```python
from build123d import *

# Parameters (mm, degrees)
SKETCH1_W            = 50
SKETCH1_H            = 88
BOSS_EXTRUDE1_DEPTH  = 0.25
BOSS_EXTRUDE2_DEPTH  = 5
SKETCH5_W            = 5
SKETCH5_H            = 11.9
BOSS_EXTRUDE3_DEPTH  = 0.05
CUT_EXTRUDE1_DEPTH   = 0.2
FILLET1_R            = 0.04
FILLET1_OF_MIRROR1_R = 0.04


with BuildPart() as part:
    # Sketch1 → Boss-Extrude1 (new body)
    with BuildSketch(Plane.XY.offset(0.25)):
        with Locations((0, 1.25)):
            Rectangle(SKETCH1_W, SKETCH1_H)
    extrude(amount=-BOSS_EXTRUDE1_DEPTH)

    # Sketch4 → Boss-Extrude2 (add)
    with BuildSketch(Plane(origin=(0, -45.25, 0), x_dir=(-1, 0, 0), z_dir=(0, -1, 0))):
        with BuildLine():
            Line((-26.45, -0.25), (26.45, -0.25))
            ThreePointArc((26.45, -0.25), (26.485355339, -0.235355339), (26.5, -0.2))
            Line((26.5, -0.2), (26.5, 1.4))
            ThreePointArc((26.5, 1.4), (26.485355339, 1.435355339), (26.45, 1.45))
            Line((26.45, 1.45), (20, 1.45))
            Line((20, 1.45), (20, 1.5))
            Line((20, 1.5), (26.5, 1.5))
            ThreePointArc((26.5, 1.5), (26.535355339, 1.485355339), (26.55, 1.45))
            Line((26.55, 1.45), (26.55, -0.25))
            ThreePointArc((26.55, -0.25), (26.535355339, -0.285355339), (26.5, -0.3))
            Line((26.5, -0.3), (-26.5, -0.3))
            ThreePointArc((-26.5, -0.3), (-26.535355339, -0.285355339), (-26.55, -0.25))
            Line((-26.55, -0.25), (-26.55, 1.45))
            ThreePointArc((-26.55, 1.45), (-26.535355339, 1.485355339), (-26.5, 1.5))
            Line((-26.5, 1.5), (-20, 1.5))
            Line((-20, 1.5), (-20, 1.45))
            Line((-20, 1.45), (-26.45, 1.45))
            ThreePointArc((-26.45, 1.45), (-26.485355339, 1.435355339), (-26.5, 1.4))
            Line((-26.5, 1.4), (-26.5, -0.2))
            ThreePointArc((-26.5, -0.2), (-26.485355339, -0.235355339), (-26.45, -0.25))
        make_face()
    boss_extrude2 = extrude(amount=-BOSS_EXTRUDE2_DEPTH)

    # Sketch5 → Boss-Extrude3 (add)
    with BuildSketch(Plane(origin=(0, 0, -1.5), x_dir=(-1, 0, 0), z_dir=(0, 0, -1))):
        with Locations((22.5, -39.3)):
            Rectangle(SKETCH5_W, SKETCH5_H)
        with Locations((-22.5, -39.3)):
            Rectangle(SKETCH5_W, SKETCH5_H)
    boss_extrude3 = extrude(amount=BOSS_EXTRUDE3_DEPTH)

    # Sketch6 → Cut-Extrude1 (cut)
    with BuildSketch(Plane(origin=(0, 0, -1.55), x_dir=(-1, 0, 0), z_dir=(0, 0, -1))):
        Polygon((20, -45.25), (25, -45.25), (20, -40.254912883), align=None)
        Polygon((-20, -40.254912883), (-25, -45.25), (-20, -45.25), align=None)
    cut_extrude1 = extrude(amount=-CUT_EXTRUDE1_DEPTH, mode=Mode.SUBTRACT)

    # Fillet1
    fillet1_edges = [part.edges().sort_by_distance(p)[0] for p in [
        (-22.5, -42.752456442, -1.45),
        (-22.5, -42.752456442, -1.55),
        (22.5, -42.752456442, -1.55),
        (22.5, -42.752456442, -1.45),
    ]]
    fillet(fillet1_edges, radius=FILLET1_R)

    # Mirror1: Boss-Extrude2, Boss-Extrude3, Cut-Extrude1 across plane
    add(boss_extrude2.mirror(Plane(origin=(0, 0, 0), x_dir=(0, 0, 1), z_dir=(0, -1, 0))))
    add(boss_extrude3.mirror(Plane(origin=(0, 0, 0), x_dir=(0, 0, 1), z_dir=(0, -1, 0))))
    add(cut_extrude1.mirror(Plane(origin=(0, 0, 0), x_dir=(0, 0, 1), z_dir=(0, -1, 0))), mode=Mode.SUBTRACT)

    # Fillet1 of Mirror1
    fillet1_of_mirror1_edges = [part.edges().sort_by_distance(p)[0] for p in [
        (-22.5, 42.752456442, -1.45),
        (-22.5, 42.752456442, -1.55),
        (22.5, 42.752456442, -1.55),
        (22.5, 42.752456442, -1.45),
    ]]
    fillet(fillet1_of_mirror1_edges, radius=FILLET1_OF_MIRROR1_R)


solid = part.part
```
Could you check a few things on this model? Use its own coordinates, in mm. Give positions to 0.01 mm unless a question says otherwise; leave off trailing zeros. Order: outer loops, then holes, each group sorted by start corner. A loop starts at its lowest first (then second) coordinate and runs counter-clockwise, first axis right, second up.
Q1. If I drill on line 1 along Z through (x, y) = (2, 16); line 2 along X through (y, z) = (20, 0.1); line 3 along Y through (x, z) = (19, 0.2), over which ranges is the centre line in solid material (lowest first)?
Q2. Suppose I cut it at C-C, the plane x = -6. Write out the boundary of the cut face in (y, z), and give its area (3 significant figures).
Q3. I'm going to push flat-ended pins straight in: P1, Ø1, axis at x = -0.5, y = -32.5, coming from the +Z side; P2, Ø1.2, axis at x = -26, y = 43.5, coming from the -Z side; P3, Ø10, axis at x = 16, y = -8, coming from the -Z side; P4, Ø1.6, axis at x = -25.5, y = -43.5, coming from the -Z side. Where does each tip first touch, or does it pass through?
Q4. Suppose I cut it at A-A, the plane z = -0.45. Write out the boundary of the cut face in (x, y), and give its area (3 significant figures).
Q5. Suppose I cut it at B-B, the plane y = 36.5. Write out the boundary of the cut face in (x, z), and give its area (3 significant figures).
Q6. Suppose I cut it at D-D, the plane x = -21.5. Count the separate pieces of the cut face and the enclosed holes in it, and give its area (3 significant figures).
Solution:
1. line 1: z = 0 to 0.25
1. line 2: x = -25 to 25
1. line 3: y = -42.75 to 45.25
2. outline: (-45.25, 0.25) - (-42.75, 0.25) - (-42.75, 0) - (45.25, 0) - (45.25, 0.3) - (40.25, 0.3) - (40.25, 0.25) - (-40.25, 0.25) - (-40.25, 0.3) - (-45.25, 0.3) - close
2. area: 22.5 mm2
3. P1: stops at z = 0.25
3. P2: stops at z = -1.5
3. P3: stops at z = 0
3. P4: stops at z = -1.55
4. outline: (-26.55, -45.25) - (-26.5, -45.25) - (-26.5, -40.25) - (-26.55, -40.25) - close; (-26.55, 40.25) - (-26.5, 40.25) - (-26.5, 45.25) - (-26.55, 45.25) - close; (26.5, -45.25) - (26.55, -45.25) - (26.55, -40.25) - (26.5, -40.25) - close; (26.5, 40.25) - (26.55, 40.25) - (26.55, 45.25) - (26.5, 45.25) - close
4. area: 1.00 mm2
5. outline: (-25, -1.55) - (-20, -1.55) - (-20, -1.5) - (-25, -1.5) - close; (-25, 0) - (25, 0) - (25, 0.25) - (-25, 0.25) - close; (20, -1.55) - (25, -1.55) - (25, -1.5) - (20, -1.5) - close
5. area: 13.0 mm2
6. separate pieces: 3
6. enclosed holes: 0
6. area: 23.5 mm2
